Read the model definition and answer for the solid it produces. Units are mm, in the model's axes. A direction names the side the tool comes from. Coordinates: 2 decimals unless noted, no trailing zeros. Write each loop counter-clockwise with the first axis right and the second up, starting at its lowest first coordinate (ties: lowest second). Pieces come first, ordered by that corner, then holes. Notation, with made-up numbers: M -11.5,-20 L 29.5,-20 A32 ccw 29.5,7 Z; hole C 88.5,1 d3. An arc over 180 degrees is marked long. Write item = value, one per line.
from build123d import *

# Parameters (mm, degrees)
BOSS_EXTRUDE1_DEPTH = 58
CUT_EXTRUDE1_DEPTH  = 90.688349299
FILLET1_R           = 2


with BuildPart() as part:
    # Sketch1 → Boss-Extrude1 (new body)
    with BuildSketch(Plane(origin=(0, 0, 0), x_dir=(1, 0, 0), z_dir=(0, 1, 0))):
        with BuildLine():
            Line((-50, -14), (36, -14))
            Line((36, -14), (36, -16))
            Line((36, -16), (-50, -16))
            ThreePointArc((-50, -16), (-61.313708499, -11.313708499), (-66, 0))
            Line((-66, 0), (-65, 0))
            ThreePointArc((-65, 0), (-64.982153791, 0.731483276), (-64.928657629, 1.461225992))
            Line((-64.928657629, 1.461225992), (-63.856406461, 2))
            ThreePointArc((-63.856406461, 2), (-60.583005244, -9.16515139), (-50, -14))
        make_face()
    extrude(amount=BOSS_EXTRUDE1_DEPTH)

    # Sketch2 → Cut-Extrude1 (cut, through all)
    with BuildSketch(Plane.XY.offset(16)):
        Polygon((36, 0), (27.714660104, 38), (7.714660104, 38), (3.353954895, 58), (36, 58), align=None)
    extrude(amount=-CUT_EXTRUDE1_DEPTH, mode=Mode.SUBTRACT)

    # Fillet1
    fillet1_edges = [part.edges().sort_by_distance(p)[0] for p in [
        (3.353954895, 58, 15),
        (27.714660104, 38, 15),
        (7.714660104, 38, 15),
        (36, 0, 15),
    ]]
    fillet(fillet1_edges, radius=FILLET1_R)


solid = part.part
Item 1: Find section D-D (y = 32). Determine the outline of the cut face in (x, z), and give its area (3 significant figures).
Worked answers:
outline = M -66,0 L -65,0 A15 ccw -64.93,-1.46 L -63.86,-2 A14 cw -50,14 L 29.02,14 L 29.02,16 L -50,16 A16 ccw Z
area = 207 mm²
Item 2: Consider line 1 along Z through (x, y) = (-30, 9); line 2 along X through (y, z) = (29, 12.5); line 3 along X through (y, z) = (8, 10.5). Determine where each line is inside the solid, lowest interval first. Write a range as from..to.
Worked answers:
line_1 = 14..16
line_2 = -59.99..-56.3
line_3 = -62.07..-59.26
Item 3: Find section B-B (x = 22). Determine the outline of the cut face in (y, z).
Worked answers:
outline = M 0,14 L 38,14 L 38,16 L 0,16 Z
Item 4: Find section C-C (z = 12). Determine the outline of the cut face in (x, y), and give its area (3 significant figures).
Worked answers:
outline = M -60.58,0 L -57.21,0 L -57.21,58 L -60.58,58 Z
area = 196 mm²
Item 5: Find section A-A (y = 6). Determine the outline of the cut face in (x, z), and give its area (3 significant figures).
Worked answers:
outline = M -66,0 L -65,0 A15 ccw -64.93,-1.46 L -63.86,-2 A14 cw -50,14 L 34.69,14 L 34.69,16 L -50,16 A16 ccw Z
area = 218 mm²
Item 6: Which of the six approach directions +Z, -Z, +X, -X, +Y, -Y give full straight-line access (tool end or side, diameter ignored) to faces 1 (the face through (-8, 29, 14)), 2 (the face through (18, 38, 15)), 3 (the face through (-19.7, 0, 14.3))?
Worked answers:
face_1 = -Z, +X, +Y, -Y
face_2 = +Z, -Z, +X, +Y
face_3 = +Z, -Z, +X, -X, -Y
Item 7: Flat-ended cylindrical pins translate along their axes: pin 1 (4 mm diameter, centred on y = 47.5, z = 4, fed in from -X); pin 2 (5 mm diameter, centred on y = 48, z = 4.5, fed in from +X); pin 3 (0.6 mm diameter, centred on x = 18.5, z = 15, fed in from +Y). Find the tip coordinate at first contact, or state that the pin passes through.
Worked answers:
pin_1 = -65.87
pin_2 = -62.12
pin_3 = 38
